```python
from build123d import *

# Parameters (mm, degrees)
F1_DEPTH = 38.1
F2_W     = 6.0325
F2_H     = 6.0325
F3_DEPTH = 19.051
F4_W     = 6.0325
F4_H     = 10.795
F5_DEPTH = 15.5575
F8_R     = 3.175


with BuildPart() as f1:
    # F0 (on Top) → F1 (new body)
    with BuildSketch(Plane.XY):
        with BuildLine():
            ThreePointArc((12.7000021839, -9.525), (22.225, 1.0919e-06), (12.7, 9.525))
            Line((12.7, 9.525), (-12.7000021839, 9.525))
            ThreePointArc((-12.7000021839, 9.525), (-22.2250021839, -1.0919e-06), (-12.7, -9.525))
            Line((-12.7, -9.525), (12.7000021839, -9.525))
        make_face()
    extrude(amount=F1_DEPTH)

    # F2 (on face) → F3 (cut, through all)
    with BuildSketch(Plane.XZ.offset(9.525)):
        with Locations((0, 19.05)):
            Rectangle(F2_W, F2_H)
    extrude(amount=-F3_DEPTH, mode=Mode.SUBTRACT)

    # F4 (on face) → F5 (cut)
    with BuildSketch(Plane.XZ.offset(9.525)):
        with Locations((0, 10.63625)):
            Rectangle(F4_W, F4_H)
    extrude(amount=-F5_DEPTH, mode=Mode.SUBTRACT)

    # F6 (on Right) → F7 (revolve, cut)
    with BuildSketch(Plane.YZ):
        Polygon((6.0325, 5.23875), (6.0325, 18.415), (-6.9215, 18.415), (-6.9215, 5.23875), (-3.6195, 5.23875), (-3.6195, 8.28675), (-0.3175, 8.28675), (-0.3175, 11.33475), (2.7305, 11.33475), (2.7305, 5.23875), align=None)
    revolve(axis=Axis((0, -0.4445, 18.415), (0, 1, 0)), mode=Mode.SUBTRACT)

    # F10: sweep along a path in F9
    with BuildLine(Plane.XZ) as f10_path:
        Line((-12.7000021839, 38.1), (-12.7000021839, 47.625))
        ThreePointArc((-12.7000021839, 47.625), (-1.0919e-06, 60.3250010919), (12.7, 47.625))
        Line((12.7, 47.625), (12.7, 41.275))
    # F8 (on face) → F10 (sweep)
    with BuildSketch(Plane.XY.offset(38.1)):
        with Locations((-12.7000021839, 0)):
            Circle(F8_R)
    sweep(path=f10_path.line)


solid = f1.part
```
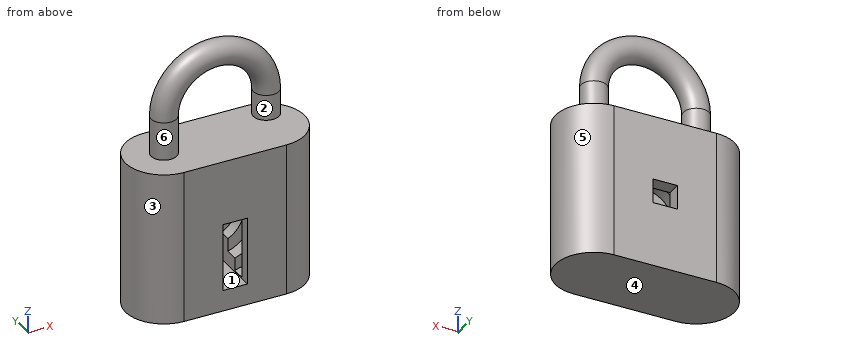
Geometry check sheet. Reference: the model listing, model coordinates, mm. Face numbers are marked on the shaded views. A direction names the side the tool comes from. Give positions to 0.01 mm unless a question says otherwise; leave off trailing zeros. Loops run counter-clockwise (first coordinate to the right, second up) from the corner with the lowest first, then second, coordinate; pieces in that order, holes last. Notation, with made-up numbers: M 9.25,6 L 68.25,6 A20 cw 68.25,42 Z; hole C 5.25,-25.5 d4. An arc over 180 degrees is marked long. Answer as CSV lines item,"result".
Item 1: Cross-section at B-B on y = 2. Record the cut outline in (x, z) (1 decimal).
Values:
outline,"M -22,0 L 22,0 L 22,38.1 L -10.2,38.1 L -10.2,47.6 A10.2 cw 10.2,47.6 L 10.2,41.3 L 15.2,41.3 L 15.2,47.6 A15.2 ccw -15.2,47.6 L -15.2,38.1 L -22,38.1 Z; hole M -3,5.2 L 3,5.2 L 3,12 A7.1 ccw long -3,12 Z"
Item 2: Cross-section at C-C on x = -4.5. Count the separate pieces of the cut face and the enclosed holes in it, and give its area (3 significant figures).
Values:
separate pieces,"2"
enclosed holes,"1"
area,"503 mm²"
Item 3: Depth check by flat-ended pin: P1, Ø6, axis at y = -2.5, z = 49.5, coming from the +X side; P2, Ø9.5, axis at x = 7, y = 2.5, coming from the +Z side; P3, Ø1.7, axis at x = -1, y = 8, coming from the +Z side. Enter the tip coordinate at first touch or a pass-through.
Values:
P1,"stops at x = 15.87"
P2,"stops at z = 63.24"
P3,"stops at z = 38.1"
Item 4: Release check for a two-part mould opening along Z. For the marked faces 4, 5 and 6 record: pulls with the +Z half, pulls with the -Z half, needs draft (parallel to the pull), parting line crosses it, or undercut.
Values:
face 4,"pulls with the -Z half"
face 5,"needs draft"
face 6,"undercut"
Item 5: Access from +Z, -Z, +X, -X, +Y, -Y to the whole of each face (thin tool, end or side, straight path). Record for the marked faces 1, 2 and 3.
Values:
face 1,"-Y"
face 2,"none"
face 3,"+Z, -Z, -X"
Item 6: Material ranges on line 1 (Y direction, x = 12, z = 19) (1 decimal); line 2 (Z direction, x = -3.5, y = -2.5); line 3 (Z direction, x = 0, y = -5.1), recorded low to high.
Values:
line 1,"y = -9.5 to -6.9, -3.6 to 2.7, 6 to 9.5"
line 2,"z = 0 to 8.91, 27.92 to 38.1, 57.78 to 61.86"
line 3,"z = 0 to 5.24, 31.59 to 38.1"
